Build history of the part. All positions in model axes, mm. Face numbers are marked on the shaded views. Round coordinates to 2 decimals unless told otherwise and drop trailing zeros. Write each loop counter-clockwise with the first axis right and the second up, starting at its lowest first coordinate (ties: lowest second). Pieces come first, ordered by that corner, then holes. Notation, with made-up numbers: (67.5, 66.25) -> (102.5, 66.25) arc R14 ccw to (102.5, 77.25) -> close; hole circle Ø2 at (-22, 34.25). An arc over 180 degrees is marked (long way). Return JSON: item names as keys, results as strings.
from build123d import *

# Parameters (mm, degrees)
BOSS_EXTRUDE1_DEPTH = 557.5
SKETCH2_W           = 50
SKETCH2_H           = 52
BOSS_EXTRUDE2_DEPTH = 323
BOSS_EXTRUDE3_DEPTH = 1115
SKETCH4_W           = 130
SKETCH4_H           = 15
CUT_EXTRUDE1_DEPTH  = 691.453655215
FILLET1_R           = 6
SKETCH8_W           = 20
SKETCH8_H           = 10
CUT_EXTRUDE3_DEPTH  = 691.453655215
SKETCH10_W          = 1065
SKETCH10_H          = 35
BOSS_EXTRUDE7_DEPTH = 13
BOSS_EXTRUDE8_DEPTH = 532.5
FILLET3_R           = 10
FILLET4_R           = 5
CHAMFER1_SIZE       = 8


with BuildPart() as part:
    # Sketch1 → Boss-Extrude1 (new, symmetric)
    with BuildSketch(Plane(origin=(0, 0, 0), x_dir=(0, 0, -1), z_dir=(1, 0, 0))):
        Polygon((0, 0), (0, 46), (52, 46), (52, 14), (15.09558328, 14), (10, 0), align=None)
    extrude(amount=BOSS_EXTRUDE1_DEPTH, both=True)

    # Sketch2 → Boss-Extrude2 (add)
    with BuildSketch(Plane(origin=(0, 46, 0), x_dir=(1, 0, 0), z_dir=(0, 1, 0))):
        with Locations((-532.5, 26)):
            Rectangle(SKETCH2_W, SKETCH2_H)
        with Locations((532.5, 26)):
            Rectangle(SKETCH2_W, SKETCH2_H)
    extrude(amount=BOSS_EXTRUDE2_DEPTH)

    # Sketch3 → Boss-Extrude3 (add)
    with BuildSketch(Plane(origin=(557.5, 0, 0), x_dir=(0, 0, -1), z_dir=(1, 0, 0))):
        Polygon((0, 369), (0, 404), (10, 404), (14.731613045, 391), (52, 391), (52, 369), align=None)
    extrude(amount=-BOSS_EXTRUDE3_DEPTH)

    # Sketch4 → Cut-Extrude1 (cut, through all)
    with BuildSketch(Plane.XY):
        with Locations((67.5, 7.5)):
            Rectangle(SKETCH4_W, SKETCH4_H)
    extrude(amount=-CUT_EXTRUDE1_DEPTH, mode=Mode.SUBTRACT)

    # Fillet1
    fillet1_edges = [part.edges().sort_by_distance(p)[0] for p in [
        (132.5, 15, -26),
        (2.5, 15, -26),
    ]]
    fillet(fillet1_edges, radius=FILLET1_R)

    # Sketch8 → Cut-Extrude3 (cut, through all)
    with BuildSketch(Plane.XY):
        with Locations((-461.5, 399)):
            Rectangle(SKETCH8_W, SKETCH8_H)
        with Locations((-385.416666667, 399)):
            Rectangle(SKETCH8_W, SKETCH8_H)
        with Locations((-309.333333333, 399)):
            Rectangle(SKETCH8_W, SKETCH8_H)
        with Locations((-233.25, 399)):
            Rectangle(SKETCH8_W, SKETCH8_H)
        with Locations((-157.166666667, 399)):
            Rectangle(SKETCH8_W, SKETCH8_H)
        with Locations((-81.083333333, 399)):
            Rectangle(SKETCH8_W, SKETCH8_H)
        with Locations((-5, 399)):
            Rectangle(SKETCH8_W, SKETCH8_H)
        with Locations((71.083333333, 399)):
            Rectangle(SKETCH8_W, SKETCH8_H)
        with Locations((147.166666667, 399)):
            Rectangle(SKETCH8_W, SKETCH8_H)
        with Locations((223.25, 399)):
            Rectangle(SKETCH8_W, SKETCH8_H)
        with Locations((299.333333333, 399)):
            Rectangle(SKETCH8_W, SKETCH8_H)
        with Locations((375.416666667, 399)):
            Rectangle(SKETCH8_W, SKETCH8_H)
        with Locations((451.5, 399)):
            Rectangle(SKETCH8_W, SKETCH8_H)
    extrude(amount=-CUT_EXTRUDE3_DEPTH, mode=Mode.SUBTRACT)

    # Sketch10 → Boss-Extrude7 (add)
    with BuildSketch(Plane(origin=(0, 0, -52), x_dir=(-1, 0, 0), z_dir=(0, 0, -1))):
        with Locations((0, 408.5)):
            Rectangle(SKETCH10_W, SKETCH10_H)
    extrude(amount=-BOSS_EXTRUDE7_DEPTH)

    # Sketch11 → Boss-Extrude8 (add, symmetric)
    with BuildSketch(Plane(origin=(0, 0, 0), x_dir=(0, 0, -1), z_dir=(1, 0, 0))):
        Polygon((39, 426), (94, 426), (94, 392), (90, 392), (83.084565549, 411), (39, 411), align=None)
    extrude(amount=BOSS_EXTRUDE8_DEPTH, both=True)

    # Fillet3
    fillet3_edges = [part.edges().sort_by_distance(p)[0] for p in [
        (0, 426, -39),
        (0, 426, -94),
    ]]
    fillet(fillet3_edges, radius=FILLET3_R)

    # Fillet4
    fillet4_edges = [part.edges().sort_by_distance(p)[0] for p in [
        (0, 411, -52),
        (0, 411, -83.084565549),
    ]]
    fillet(fillet4_edges, radius=FILLET4_R)

    # Chamfer1
    chamfer1_edges = [part.edges().sort_by_distance(p)[0] for p in [
        (0, 46, 0),
        (0, 46, -52),
        (0, 369, -52),
        (0, 369, 0),
    ]]
    chamfer(chamfer1_edges, length=CHAMFER1_SIZE)


solid = part.part
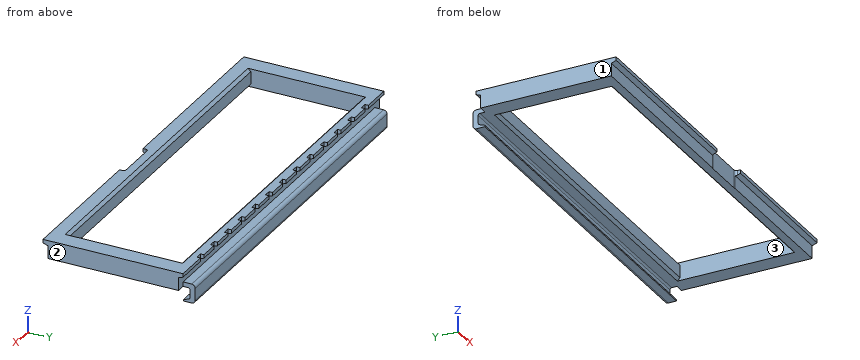
Q1. Two-plate mould, pull along X, no slides. Class the marked faces 1, 2 and 3: +X half, -X half, draft (parallel to the pull), parting line (faces both ways), or undercut.
Verdict:
{"face 1": "-X half", "face 2": "+X half", "face 3": "undercut"}
Q2. Pin check, flat tips, straight feed: pin 1 Ø11 at (x, z) = (220, -5.5) entering from +Y; pin 2 Ø12 at (x, z) = (153.5, -55.5) entering from -Y; pin 3 Ø5 at (x, z) = (-429, -4.5) entering from +Y; pin 4 Ø12 at (x, y) = (157.5, 57.5) entering from -Z. Stop position of each tip, or through.
Verdict:
{"pin 1": "stops at y = 394", "pin 2": "stops at y = 14", "pin 3": "stops at y = 404", "pin 4": "passes through"}
Q3. Saw through at B-B on y = 91. List the corners of the cut face in (x, z).
Verdict:
{"outline": "(-557.5, -52) -> (-507.5, -52) -> (-507.5, 0) -> (-557.5, 0) -> close; (507.5, -52) -> (557.5, -52) -> (557.5, 0) -> (507.5, 0) -> close"}
Q4. Wall check: L1, parallel to Y at x = 493.5, z = -23; L2, parallel to X at y = 272, z = -34.5; L3, parallel to Z at x = 348, y = 393. Give the ranges that are in metal, low to high.
Verdict:
{"L1": "y = 14 to 46, 369 to 391", "L2": "x = -557.5 to -507.5, 507.5 to 557.5", "L3": "z = -94 to -89.64, -52 to -39, -14 to 0"}
Q5. Saw through at A-A on x = 49. List the corners of the cut face in (y, z), then the cut area to 3 significant figures.
Verdict:
{"outline": "(15, -52) -> (38, -52) -> (46, -44) -> (46, -8) -> (38, 0) -> (15, 0) -> close; (369, -44) -> (377, -52) -> (406, -52) arc R5 cw to (411, -57) -> (411, -79.58) arc R5 cw to (407.71, -84.28) -> (392, -90) -> (392, -94) -> (416, -94) arc R10 ccw to (426, -84) -> (426, -49) arc R10 ccw to (416, -39) -> (391, -39) -> (391, -14.73) -> (404, -10) -> (404, 0) -> (377, 0) -> (369, -8) -> close", "area": "3,980 mm²"}
Q6. Saw through at C-C on x = -486.5. List the corners of the cut face in (y, z).
Verdict:
{"outline": "(0, -10) -> (14, -15.1) -> (14, -52) -> (38, -52) -> (46, -44) -> (46, -8) -> (38, 0) -> (0, 0) -> close; (369, -44) -> (377, -52) -> (406, -52) arc R5 cw to (411, -57) -> (411, -79.58) arc R5 cw to (407.71, -84.28) -> (392, -90) -> (392, -94) -> (416, -94) arc R10 ccw to (426, -84) -> (426, -49) arc R10 ccw to (416, -39) -> (391, -39) -> (391, -14.73) -> (404, -10) -> (404, 0) -> (377, 0) -> (369, -8) -> close"}
